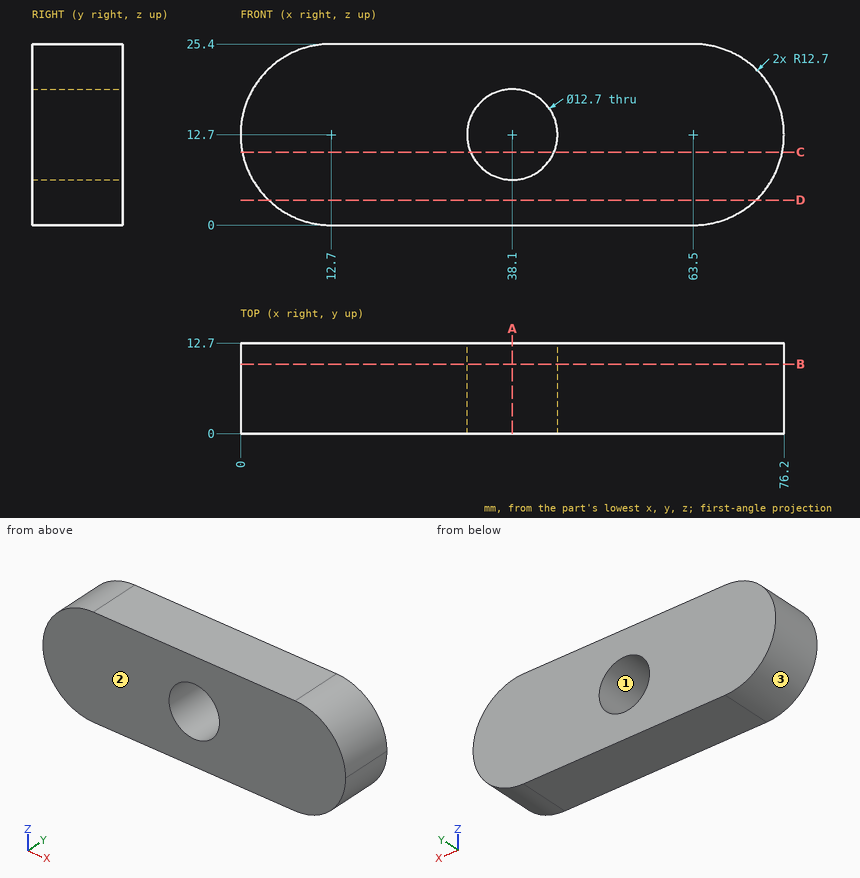
Print and shaded views of the part. All mm, measured from the part's lowest x, y and z. Round coordinates to 2 decimals unless told otherwise and drop trailing zeros. Write each loop counter-clockwise with the first axis right and the second up, starting at its lowest first coordinate (ties: lowest second). Pieces come first, ordered by that corner, then holes. Notation, with made-up numbers: (-18, -40) - (25, -40) arc R15 cw to (25, -23) - close; hole circle Ø2 at (4.5, 13.25). An arc over 180 degrees is marked (long way). One line per question, with ' | ' between items.
1. Drop flat-ended pins along their axis: pin 1 Ø3 at (y, z) = (7, 5.5) entering from -X; pin 2 Ø2 at (y, z) = (11, 3.5) entering from -X; pin 3 Ø5 at (x, y) = (67, 9) entering from +Z. Give the stop position or say it passes through.
Results are:
pin 1: x = 1.35 | pin 2: x = 3 | pin 3: z = 25.36
2. Band-saw the part on B-B, the plane y = 9.75. Write the cut outline in (x, z).
Results are:
outline: (12.7, 0) - (63.5, 0) arc R12.7 ccw to (63.5, 25.4) - (12.7, 25.4) arc R12.7 ccw to start; hole circle Ø12.7 at (38.1, 12.7)
3. Band-saw the part on D-D, the plane z = 3.5. Write the cut outline in (x, y) (3 decimals).
Results are:
outline: (3.945, 0) - (72.255, 0) - (72.255, 12.7) - (3.945, 12.7) - close
4. Mould opens along X. For the marked faces 1, 2 and 3 say: released by +X, released by -X, zero draft, split by the parting line, or undercut.
Results are:
face 1: undercut | face 2: zero draft | face 3: released by -X
5. Band-saw the part on C-C, the plane z = 10.25. Write the cut outline in (x, y).
Results are:
outline: (0.24, 0) - (32.24, 0) - (32.24, 12.7) - (0.24, 12.7) - close; (43.96, 0) - (75.96, 0) - (75.96, 12.7) - (43.96, 12.7) - close
6. Band-saw the part on A-A, the plane x = 38.1. Write the cut outline in (y, z).
Results are:
outline: (0, 0) - (12.7, 0) - (12.7, 6.35) - (0, 6.35) - close; (0, 19.05) - (12.7, 19.05) - (12.7, 25.4) - (0, 25.4) - close
7. Drill centre lines: line 1 along Z through (x, y) = (38.1, 4.75); line 2 along X through (y, z) = (6.5, 17); line 3 along X through (y, z) = (8, 18.5). Where is each one in solid material? Low to high. Write a range as from..to.
Results are:
line 1: 0..6.35, 19.05..25.4 | line 2: 0.75..33.43, 42.77..75.45 | line 3: 1.4..35.51, 40.69..74.8
